Design review of the part built by this model. Coordinates are the model's own, in mm. A direction names the side the tool comes from. Give positions to 0.01 mm unless a question says otherwise; leave off trailing zeros. Order: outer loops, then holes, each group sorted by start corner. A loop starts at its lowest first (then second) coordinate and runs counter-clockwise, first axis right, second up. Notation, with made-up numbers: (31, -3.75) - (77, -3.75) arc R14 cw to (77, 13.25) - close; hole circle Ø10 at (37.5, 79). An arc over 180 degrees is marked (long way). Write each question's results on one line, items separated by ' | '. Start each with the question number.
```python
from build123d import *

# Parameters (mm, degrees)
ESQUISSE1_W                                        = 40
ESQUISSE1_H                                        = 11
ESQUISSE1_R                                        = 4
BOSS_EXTRU_1_DEPTH                                 = 10.51
ESQUISSE16_W                                       = 40
ESQUISSE16_H                                       = 11
BOSS_EXTRU_2_DEPTH                                 = 7
D_GAGEMENT_M32_D                                   = 2.5
CHAMBRAGE_POUR_VIS_T_TE_RONDE_BOMB_E_M_D           = 3.4
CHAMBRAGE_POUR_VIS_T_TE_RONDE_BOMB_E_M_CBORE_D     = 6
CHAMBRAGE_POUR_VIS_T_TE_RONDE_BOMB_E_M_CBORE_DEPTH = 2.4
FRAISAGE_POUR_VIS_T_TE_FRAIS_E_M31_D               = 3.4
FRAISAGE_POUR_VIS_T_TE_FRAIS_E_M31_DEPTH           = 8
FRAISAGE_POUR_VIS_T_TE_FRAIS_E_M31_CSINK_D         = 6.3
FRAISAGE_POUR_VIS_T_TE_FRAIS_E_M31_CSINK_ANGLE     = 90
FRAISAGE_POUR_VIS_T_TE_FRAIS_E_M31_TIP             = 1.021463052
ESQUISSE33_W                                       = 100.854971174
ESQUISSE33_H                                       = 90.146734576
ENL_V_MAT_EXTRU_4_DEPTH                            = 3
ESQUISSE34_R                                       = 4
ENL_V_MAT_EXTRU_5_DEPTH                            = 10
ESQUISSE35_W                                       = 78.795727906
ESQUISSE35_H                                       = 40.956962542
ENL_V_MAT_EXTRU_6_DEPTH                            = 3


with BuildPart() as part:
    # Esquisse1 → Boss.-Extru.1 (new body)
    with BuildSketch(Plane.XY):
        Rectangle(ESQUISSE1_W, ESQUISSE1_H)
        Circle(ESQUISSE1_R, mode=Mode.SUBTRACT)
    extrude(amount=BOSS_EXTRU_1_DEPTH)

    # Esquisse16 → Boss.-Extru.2 (add)
    with BuildSketch(Plane.XY.offset(10.51)):
        Rectangle(ESQUISSE16_W, ESQUISSE16_H)
    extrude(amount=BOSS_EXTRU_2_DEPTH)

    # Dégagement M32 (through all)
    with Locations(Plane.XY.offset(17.51)):
        with Locations((0, 0)):
            Hole(D_GAGEMENT_M32_D / 2)

    # Chambrage pour vis _ t_te ronde bomb_e M (through all)
    with Locations(Plane(origin=(0, 5.5, 0), x_dir=(1, 0, 0), z_dir=(0, 1, 0))):
        with Locations((10, -9.51), (-10, -9.51)):
            CounterBoreHole(CHAMBRAGE_POUR_VIS_T_TE_RONDE_BOMB_E_M_D / 2, CHAMBRAGE_POUR_VIS_T_TE_RONDE_BOMB_E_M_CBORE_D / 2, CHAMBRAGE_POUR_VIS_T_TE_RONDE_BOMB_E_M_CBORE_DEPTH)

    # Fraisage pour vis à tête fraisée M31
    with Locations(Plane.XY.offset(17.51)):
        with Locations((-15, 0), (15, 0)):
            CounterSinkHole(FRAISAGE_POUR_VIS_T_TE_FRAIS_E_M31_D / 2, FRAISAGE_POUR_VIS_T_TE_FRAIS_E_M31_CSINK_D / 2, depth=FRAISAGE_POUR_VIS_T_TE_FRAIS_E_M31_DEPTH, counter_sink_angle=FRAISAGE_POUR_VIS_T_TE_FRAIS_E_M31_CSINK_ANGLE)
            with Locations((0, 0, -(FRAISAGE_POUR_VIS_T_TE_FRAIS_E_M31_DEPTH + FRAISAGE_POUR_VIS_T_TE_FRAIS_E_M31_TIP / 2))):  # 118° drill point
                Cone(0, FRAISAGE_POUR_VIS_T_TE_FRAIS_E_M31_D / 2, FRAISAGE_POUR_VIS_T_TE_FRAIS_E_M31_TIP, mode=Mode.SUBTRACT)

    # Esquisse33 → Enlèv. mat.-Extru.4 (cut)
    with BuildSketch(Plane.XY.offset(17.51)):
        Rectangle(ESQUISSE33_W, ESQUISSE33_H)
    extrude(amount=-ENL_V_MAT_EXTRU_4_DEPTH, mode=Mode.SUBTRACT)

    # Esquisse34 → Enlèv. mat.-Extru.5 (cut)
    with BuildSketch(Plane.XY.offset(14.51)):
        Circle(ESQUISSE34_R)
    extrude(amount=-ENL_V_MAT_EXTRU_5_DEPTH, mode=Mode.SUBTRACT)

    # Esquisse35 → Enlèv. mat.-Extru.6 (cut)
    with BuildSketch(Plane(origin=(0, 0, 0), x_dir=(-1, 0, 0), z_dir=(0, 0, -1))):
        Rectangle(ESQUISSE35_W, ESQUISSE35_H)
    extrude(amount=-ENL_V_MAT_EXTRU_6_DEPTH, mode=Mode.SUBTRACT)


solid = part.part
```
Q1. Add section C-C (z = 10.25). Give the boundary of the cut face in (x, y), plus the area to 3 significant figures.
Q2. Add section B-B (y = -3). Give the boundary of the cut face in (x, z), plus the area to 3 significant figures.
Q3. For line 1 (X direction, y = 0, z = 12.4); line 2 (X direction, y = 0, z = 5.5); line 3 (Y direction, x = -15, z = 11), list the stretches that pass through material, from the lowest coordinate up. Write a range as [from, to].
Q4. Add section A-A (x = 10). Give the boundary of the cut face in (y, z), plus the area to 3 significant figures.
Q5. Insertion check: pin 1 Ø5 at (x, z) = (10, 9.51) entering from +Y; pin 2 Ø5 at (x, z) = (8.5, 8) entering from +Y. Each pin has a flat end and moves straight along its axis. Give the tip position at first contact, or say it passes through.
Q6. Add section D-D (y = 5). Give the boundary of the cut face in (x, z).
Q7. Machinability: for faces 4 (the flat face through (0, 5.5, 9)), 5 (the cylindrical face through (13.38, 0.51, 11.98)), 6 (the cylindrical face through (11.61, 4.32, 6.98)), which of the approach directions +Z, -Z, +X, -X, +Y, -Y give a long, thin tool a straight path to every point of the face, cutting with its end or side? Answer none if there is none.
Q8. Draft analysis for pull direction Z (two halves, no side actions). For faces 1 (the cylindrical face through (-0.867, -3.905, 8.674)), 2 (the flat face through (-8, 3.1, 9)), 3 (the conical face through (15.282, 0.089, 8.666)), state which applies: pulls with the +Z half, pulls with the -Z half, needs draft (parallel to the pull), parting line crosses it, or undercut.
Verdict:
1) outline: (-20, -5.5) - (-11.53, -5.5) - (-11.53, 3.1) - (-12.91, 3.1) - (-12.91, 5.5) - (-20, 5.5) - close; (-8.47, -5.5) - (8.47, -5.5) - (8.47, 3.1) - (7.09, 3.1) - (7.09, 5.5) - (-7.09, 5.5) - (-7.09, 3.1) - (-8.47, 3.1) - close; (11.53, -5.5) - (20, -5.5) - (20, 5.5) - (12.91, 5.5) - (12.91, 3.1) - (11.53, 3.1) - close; hole circle Ø3.4 at (-15, 0); hole circle Ø8 at (0, 0); hole circle Ø3.4 at (15, 0) | area: 291 mm2
2) outline: (-20, 3) - (-2.65, 3) - (-2.65, 14.51) - (-20, 14.51) - close; (2.65, 3) - (20, 3) - (20, 14.51) - (2.65, 14.51) - close; hole circle Ø3.4 at (-10, 9.51); hole circle Ø3.4 at (10, 9.51) | area: 381 mm2
3) line 1: x = [-20, -16.7], [-13.3, -4], [4, 13.3], [16.7, 20] | line 2: x = [-20, -4], [4, 20] | line 3: y = [-5.5, -1.7], [1.7, 5.5]
4) outline: (-5.5, 3) - (5.5, 3) - (5.5, 6.51) - (3.1, 6.51) - (3.1, 7.81) - (-5.5, 7.81) - close; (-5.5, 11.21) - (3.1, 11.21) - (3.1, 12.51) - (5.5, 12.51) - (5.5, 14.51) - (-5.5, 14.51) - close | area: 83.0 mm2
5) pin 1: stops at y = 3.1 | pin 2: stops at y = 5.5
6) outline: (-20, 3) - (20, 3) - (20, 14.51) - (-20, 14.51) - close; hole circle Ø6 at (-10, 9.51); hole circle Ø6 at (10, 9.51)
7) face 4: +Z, -Z, +X, -X, +Y | face 5: +Z | face 6: +Y
8) face 1: needs draft | face 2: undercut | face 3: pulls with the +Z half
